The model under review builds one solid part; all positions refer to its coordinate system, in mm. A direction names the side the tool comes from. Coordinates: 2 decimals unless noted, no trailing zeros. Write each loop counter-clockwise with the first axis right and the second up, starting at its lowest first coordinate (ties: lowest second). Pieces come first, ordered by that corner, then holes. Notation, with made-up numbers: (-36, 45.5) - (-27, 45.5) arc R32 ccw to (-27, 84.5) - close; hole circle Ø1 at (68.5, 45.5). An arc over 180 degrees is marked (long way). Put each result on its own line as item: value. Start each with the question number.
Item 1: Consider section C-C on y = -22. Give the boundary of the cut face in (x, z).
Item 2: For pin 1 (0.8 mm diameter, centred on x = -40.5, z = -19, fed in from -Y); pin 2 (2 mm diameter, centred on x = -9.5, y = -6, fed in from +Z); pin 3 (10 mm diameter, centred on y = 10.5, z = -7, fed in from +X); pin 4 (0.9 mm diameter, centred on x = -26.5, y = 3, fed in from -Z), all flat-tipped, find the tip position at first contact; note any pin that passes through.
Item 3: Machinability: for faces 1 (the face through (-14, 0, -10)), 2 (the face through (-1.5, 10, -1)), 3 (the face through (-38, 0, -19)), 4 (the face through (9, -23, -2.75)), 5 (the face through (-30, 3, -2)), which of the approach directions +Z, -Z, +X, -X, +Y, -Y give a long, thin tool a straight path to every point of the face, cutting with its end or side? Answer none if there is none.
Item 4: Mouldability with a two-part tool opening along Y and no side actions: class faces 6 (the face through (12.8, 9.4, -27.5)), 7 (the face through (8, 0, -27)), 8 (the face through (-15, 19, -18)), 9 (the face through (-30, 3, -18)) as pulls with the +Y half, pulls with the -Y half, needs draft (parallel to the pull), parting line crosses it, or undercut.
Item 5: Consider section D-D on x = 18. Give the boundary of the cut face in (y, z), then the cut area to 3 significant figures.
Item 6: Consider section B-B on x = -44. Give the boundary of the cut face in (y, z), then the cut area to 3 significant figures.
Item 7: To check wall thickness, follow L1, parallel to Z at x = -20.5, y = 2; L2, parallel to Z at x = -12, y = -13.5; L3, parallel to X at y = 13.5, z = -1.5. State the ranges of each line that lie inside material, in increasing order. Write a range as [from, to].
Item 8: Consider section A-A on z = -15. Give the boundary of the cut face in (x, y).
Autodesk Inventor part; units mm, degrees
ref_plane "YZ Plane" through (0, 0, 0) normal (1, 0, 0) x (0, 1, 0)
ref_plane "XZ Plane" through (0, 0, 0) normal (0, 1, 0) x (-1, 0, 0)
ref_plane "XY Plane" through (0, 0, 0) normal (0, 0, 1) x (1, 0, 0)
sketch "Sketch1" plane through (0, 0, 0) normal (0, 1, 0) x (-1, 0, 0)
  line L0 (0, 0) -> (60, 0)
  line L1 (60, 0) -> (60, -20)
  line L2 (60, -20) -> (0, -20)
  line L3 (0, -20) -> (0, 0)
  dimension "d0" = 60
  dimension "d1" = 20
extrude "Extrusion1" add sketch "Sketch1" along normal blind 5
sketch "Sketch2" plane through (0, 5, 0) normal (0, 1, 0) x (1, 0, 0)
  line L0 (0, 20) -> (-60, 20)
  line L1 (0, 0) -> (0, 20)
  line L2 (-60, 20) -> (0, 20)
  line L3 (0, 20) -> (0, 17.5)
  line L4 (0, 17.5) -> (-60, 17.5)
  line L5 (-60, 17.5) -> (-60, 20)
  line L6 (-60, 20) -> (-60, 0)
  line L7 (-60, 0) -> (0, 0)
  line L8 (0, 0) -> (0, 2.5)
  line L9 (0, 2.5) -> (-60, 2.5)
  line L10 (-60, 2.5) -> (-60, 0)
  line L11 (-60, 0) -> (0, 0)
  line L12 (-60, 20) -> (-57.5, 20)
  line L13 (-57.5, 20) -> (-57.5, 0)
  line L14 (-57.5, 0) -> (-60, 0)
  line L15 (-60, 0) -> (-60, 20)
  line L16 (0, 20) -> (-2, 20)
  line L17 (-2, 20) -> (-2, 17.5)
  line L18 (-2, 17.5) -> (0, 17.5)
  line L19 (0, 17.5) -> (0, 20)
  line L20 (0, 2.5) -> (-2, 2.5)
  line L21 (-2, 2.5) -> (-2, 0)
  line L22 (-2, 0) -> (0, 0)
  line L23 (0, 0) -> (0, 2.5)
  point P0 (0, 2.5)
  point P1 (-57.5, 2.5)
  point P2 (-57.5, 17.5)
  dimension "d4" = 2.5
  dimension "d5" = 2.5
  dimension "d6" = 2.5
  dimension "d9" = 15
  dimension "d20" = 2
extrude "Extrusion2" add sketch "Sketch2" along normal blind 14 contours L1 L4 L17 L0 | L17 L4 L13 L0 | L13 L4 L5 L0 | L1 L7 L21 L9 | L13 L9 L6 L4 | L21 L7 L13 L9 | L13 L7 L6 L9
sketch "Sketch3" plane through (0, 5, 0) normal (0, 1, 0) x (1, 0, 0)
  line L0 (0, 0) -> (0, 2.5)
  line L1 (0, 0) -> (26, 0)
  line L2 (26, 0) -> (26, 20)
  line L3 (26, 20) -> (0, 20)
  line L4 (0, 20) -> (0, 0)
  circle A0 centre (13, 10) radius 17.5
  circle A1 centre (13, 10) radius 20
  line L5 (0, 2.5) -> (-57.5, 2.5)
  line L6 (0, 2.5) -> (26, 2.5)
  line L7 (26, 2.5) -> (26, 17.5)
  line L8 (26, 17.5) -> (0, 17.5)
  line L9 (0, 17.5) -> (0, 2.5)
  line L10 (0, 17.5) -> (-57.5, 17.5)
  line L11 (-57.5, 17.5) -> (-57.5, 2.5)
  line L12 (-57.5, 2.5) -> (0, 2.5)
  line L13 (0, 2.5) -> (0, 17.5)
  line L14 (-5.5405, 2.5) -> (0, 2.5)
  line L15 (-60, 0) -> (0, 0)
  line L16 (0, 0) -> (0, 2.5)
  line L17 (0, 2.5) -> (-57.5, 2.5)
  line L18 (-57.5, 2.5) -> (-57.5, 17.5)
  line L19 (-57.5, 17.5) -> (0, 17.5)
  line L20 (0, 17.5) -> (0, 20)
  line L21 (0, 20) -> (-60, 20)
  line L22 (-60, 20) -> (-60, 0)
  line L23 (-5.5405, 17.5) -> (0, 17.5)
  line L24 (26, 17.5) -> (31.5405, 17.5)
  line L25 (26, 2.5) -> (31.5405, 2.5)
  line L26 (26, 20) -> (30.3205, 20)
  line L27 (26, 0) -> (30.3205, 0)
  point P0 (-4.3205, 20)
  point P1 (-1.3614, 20)
  point P2 (-1.3614, 0)
  point P3 (-4.3205, 0)
  point P4 (28.8114, 2.5)
  point P5 (28.8114, 17.5)
  point P6 (27.3614, 20)
  point P7 (27.3614, 0)
  dimension "d10" = 26
  dimension "d11" = 20
  dimension "d13" = 35
  dimension "d14" = 40
  dimension "d17" = 15
extrude "Extrusion3" add sketch "Sketch3" along normal blind 14 and the other way blind 5 contours A0 L27 A1 L15 | L21 A1 L26 A0
sketch "Sketch4" plane through (0, 0, 0) normal (0, -1, 0) x (1, 0, 0)
  point P0 (0, 0)
sketch "Sketch5" plane through (0, 0, 0) normal (1, 0, 0) x (0, 0, -1)
  line L0 (17.5, 19) -> (20, 19)
  line L1 (0, 0) -> (20, 0)
  line L2 (20, 19) -> (17.5, 19)
  line L3 (17.5, 19) -> (17.5, 0)
  line L4 (17.5, 0) -> (20, 0)
  line L5 (20, 0) -> (20, 19)
  line L6 (2.5, 5) -> (2.5, 19)
  line L7 (2.5, 19) -> (0, 19)
  line L8 (0, 19) -> (0, 0)
  line L9 (0, 0) -> (2.5, 0)
  line L10 (2.5, 0) -> (2.5, 19)
  line L11 (17.5, 5) -> (2.5, 5)
  line L12 (2.5, 5) -> (2.5, 0)
  line L13 (2.5, 0) -> (17.5, 0)
  line L14 (17.5, 0) -> (17.5, 5)
  dimension "d21" = 2.5
extrude "Extrusion4" cut sketch "Sketch5" against normal blind 1.5
sketch "Sketch7" plane through (-60, 0, 0) normal (0, 0, 1) x (1, 0, 0)
  line L0 (0, 0) -> (55.6795, 0)
  line L1 (55.6795, 0) -> (90.3205, 0)
  line L2 (55.6795, 0) -> (55.6795, 19)
  line L3 (55.6795, 0) -> (48.6795, 0)
  line L4 (48.6795, 0) -> (48.6795, -25)
  line L5 (48.6795, -25) -> (55.6795, -25)
  line L6 (55.6795, -25) -> (55.6795, 0)
  line L7 (55.6795, -25) -> (90.6795, -25)
  line L8 (90.6795, -25) -> (90.6795, -20)
  line L9 (90.6795, -20) -> (55.6795, -20)
  line L10 (55.6795, -20) -> (55.6795, -25)
  point P0 (60, 0)
  dimension "d25" = 7
  dimension "d26" = 25
  dimension "d27" = 35
  dimension "d28" = 5
extrude "Extrusion5" add sketch "Sketch7" against normal up to surface (20 mm away)
sketch "Sketch8" plane through (0, 0, 0) normal (0, -1, 0) x (1, 0, 0)
  point P0 (0, 0)
sketch "Sketch9" plane through (-11.3205, -25, 0) normal (0, -1, 0) x (1, 0, 0)
  line L0 (0, -20) -> (42, -20)
  line L1 (0, 0) -> (42, 0)
  arc A0 (7, -20) -> (41.641, -20) centre (24.3205, -10) ccw
  line L2 (42.861, -17.5) -> (40.1319, -17.5)
  arc A1 (9.9591, -20) -> (38.6819, -20) centre (24.3205, -10) ccw
  line L3 (9.9591, -20) -> (9.8205, -20)
  line L4 (9.8205, 0) -> (9.9591, 0)
  arc A2 (38.6819, 0) -> (9.9591, 0) centre (24.3205, -10) ccw
  line L5 (40.1319, -2.5) -> (42.861, -2.5)
  arc A3 (41.641, 0) -> (7, 0) centre (24.3205, -10) ccw
  line L6 (5, -2.75) -> (40, -2.75)
  line L7 (40, -2.75) -> (40, -17.25)
  line L8 (40, -17.25) -> (5, -17.25)
  line L9 (5, -17.25) -> (5, -2.75)
  line L10 (0, 0) -> (0, -20)
  point P0 (11.3205, 0)
  point P1 (5, -10)
  dimension "d36" = 35
  dimension "d37" = 14.5
  dimension "d38" = 5
  dimension "d39" = 2.75
extrude "Extrusion6" cut sketch "Sketch9" against normal blind 10 contours L6 L7 L8 L9
sketch "Sketch10" plane through (-1.5, 0, 0) normal (1, 0, 0) x (0, 0, -1)
  line L0 (2.5, 5) -> (17.5, 5)
  line L1 (2.5, 19) -> (2.5, 5)
  line L2 (17.5, 5) -> (17.5, 19)
  line L3 (20, 0) -> (0, 0)
  line L4 (2.5, 5) -> (17.5, 5)
  line L5 (17.5, 5) -> (17.5, 0)
  line L6 (17.5, 0) -> (2.5, 0)
  line L7 (2.5, 0) -> (2.5, 5)
  line L8 (2.5, 4) -> (2, 4)
  line L9 (2, 4) -> (2, 1)
  line L10 (2, 1) -> (2.5, 1)
  line L11 (2.5, 1) -> (2.5, 4)
  line L12 (0, 0) -> (0, 19)
  line L13 (17.5, 4) -> (18, 4)
  line L14 (18, 4) -> (18, 1)
  line L15 (18, 1) -> (17.5, 1)
  line L16 (17.5, 1) -> (17.5, 4)
  line L17 (20, 19) -> (20, 0)
  point P0 (2.25, 4)
  point P1 (2.25, 1)
  point P2 (18, 2.5)
  point P3 (17.75, 1)
  point P4 (17.75, 4)
  point P5 (17.5, 1)
  point P6 (2.5, 1)
  dimension "d42" = 2
  dimension "d43" = 1
  dimension "d44" = 1
  dimension "d45" = 2
  dimension "d46" = 1
  dimension "d47" = 1
  dimension "d49" = 2.5
extrude "Extrusion7" cut sketch "Sketch10" against normal through all
sketch "Sketch11" plane through (-11.3205, -25, 0) normal (-1, 0, 0) x (0, 0, 1)
  line L0 (0, 25) -> (0, 0)
  line L1 (-20, 25) -> (-20, 0)
  line L2 (0, 0) -> (-20, 0)
  line L3 (-20, 0) -> (-20, 25)
  line L4 (-20, 25) -> (0, 25)
  line L5 (0, 25) -> (0, 0)
extrude "Extrusion8" add sketch "Sketch11" along normal blind 5
sketch "Sketch12" plane through (-4.3205, -20, 0) normal (1, 0, 0) x (0, 0, -1)
  line L0 (2.75, 5) -> (17.25, 5)
  line L1 (17.25, 0) -> (20, 0)
  line L2 (17.25, 5) -> (20, 5)
  line L3 (20, 5) -> (20, 0)
  line L4 (20, 0) -> (17.25, 0)
  line L5 (17.25, 0) -> (17.25, 5)
  line L6 (2.75, -5) -> (2.75, 5)
  line L7 (0, -5) -> (0, 20)
  line L8 (2.75, 5) -> (0, 5)
  line L9 (0, 5) -> (0, 0)
  line L10 (0, 0) -> (2.75, 0)
  line L11 (2.75, 0) -> (2.75, 5)
  line L12 (0, 20) -> (2.5, 20)
  line L13 (20, 5) -> (0, 5)
  line L14 (0, 5) -> (0, 20)
  line L15 (0, 20) -> (20, 20)
  line L16 (20, 20) -> (20, 5)
  point P0 (2.75, 0)
extrude "Extrusion9" cut sketch "Sketch12" against normal blind 7
sketch "Sketch13" plane through (-6.3205, -25, -2.75) normal (1, 0, 0) x (0, 0, -1)
  line L0 (0, 0) -> (0, 5)
  line L1 (14.5, 10) -> (0, 10)
  line L2 (0, 10) -> (0, 0)
  line L3 (0, 0) -> (14.5, 0)
  line L4 (14.5, 0) -> (14.5, 10)
  point P0 (-2.75, 25)
  point P1 (0, 5)
extrude "Extrusion10" cut sketch "Sketch13" against normal blind 5
sketch "Sketch14" plane through (-1.5, 19, -2.5) normal (0, 0, -1) x (-1, 0, 0)
  point P0 (-1.5, -19)
properties part number "Magasin_3DPrint"
Report:
1. outline: (-16.32, -20) - (30.68, -20) - (30.68, 0) - (-16.32, 0) - close; hole (-11.32, -17.25) - (28.68, -17.25) - (28.68, -2.75) - (-11.32, -2.75) - close
2. pin 1: y = 0
2. pin 2: through
2. pin 3: x = -1.5
2. pin 4: z = -20
3. face 1: +X, -X, +Y
3. face 2: +X, +Y
3. face 3: +Z, -Z, -X, -Y
3. face 4: +Y, -Y
3. face 5: +X, -X
4. face 6: needs draft
4. face 7: undercut
4. face 8: pulls with the +Y half
4. face 9: undercut
5. outline: (-25, -20) - (-20, -20) - (-20, -17.25) - (-25, -17.25) - close; (-25, -2.75) - (-20, -2.75) - (-20, 0) - (-25, 0) - close; (0, -29.36) - (19, -29.36) - (19, -26.77) - (0, -26.77) - close; (0, 6.77) - (19, 6.77) - (19, 9.36) - (0, 9.36) - close
5. area: 126 mm²
6. outline: (0, -20) - (19, -20) - (19, -17.5) - (4, -17.5) - (4, -18) - (1, -18) - (1, -17.5) - (0, -17.5) - close; (0, -2.5) - (1, -2.5) - (1, -2) - (4, -2) - (4, -2.5) - (19, -2.5) - (19, 0) - (0, 0) - close
6. area: 92.0 mm²
7. L1: [-20, -18], [-2, 0]
7. L2: [-20, 0]
7. L3: [-60, -1.5]
8. outline: (-60, 5) - (-57.5, 5) - (-57.5, 19) - (-60, 19) - close; (-16.32, -25) - (-11.32, -25) - (-11.32, 0) - (-16.32, 0) - close; (28.68, -25) - (30.68, -25) - (30.68, -20) - (28.68, -20) - close
